```python
from build123d import *

# Parameters (mm, degrees)
BOSS_EXTRUDE1_DEPTH     = 15
SCALE1_SCALE            = 0.6
CUT_EXTRUDE2_DEPTH      = 414.628802078
CUT_EXTRUDE2_DEPTH_BACK = 414.628802078


with BuildPart() as part:
    # Sketch3 → Boss-Extrude1 (new body)
    with BuildSketch(Plane.XY):
        Polygon((373.374123275, 416.968077367), (402.437373481, 34.910153282), (374.539751445, 1.298077367), (346.074948764, 1.298077367), (346.074948764, 416.968077367), align=None)
    extrude(amount=BOSS_EXTRUDE1_DEPTH)


with BuildPart() as part_1:
    # Scale1: scaled about (367.849283485, 188.760033588, 7.5)
    add(part.part.scale(SCALE1_SCALE).moved(Location((147.139713394, 75.504013435, 3))))

    # Sketch9 → Cut-Extrude2 (cut, two sides: drawn at the far end of the back side and taken through both)
    with BuildSketch(Plane(origin=(0, 184.5, 0), x_dir=(1, 0, 0), z_dir=(0, 1, 0)).offset(-CUT_EXTRUDE2_DEPTH_BACK)):
        with BuildLine():
            Line((354.784682653, -12), (354.784682653, -3))
            ThreePointArc((354.784682653, -3), (356.648643683, -7.5), (354.784682653, -12))
        make_face()
    extrude(amount=CUT_EXTRUDE2_DEPTH + CUT_EXTRUDE2_DEPTH_BACK, mode=Mode.SUBTRACT)


solid = part_1.part
```
The listing builds one solid part. Answer for the finished solid, in the listing's coordinates (mm). Round coordinates to 2 decimals unless told otherwise and drop trailing zeros. Order: outer loops, then holes, each group sorted by start corner. A loop starts at its lowest first (then second) coordinate and runs counter-clockwise, first axis right, second up. Notation, with made-up numbers: (47, -22) -> (55, -22) arc R12 ccw to (55, -5) -> close; hole circle Ø8 at (-26.75, -10). An arc over 180 degrees is marked (long way). Answer as CSV lines item,"result". Start each with the question number.
(1) Find the intervals of material crossed by probe 1 along X at (y, z) = (130, 8.5); probe 2 along X at (y, z) = (311.5, 4.75), in increasing order. Write a range as from..to.
(2) Flat-ended cylindrical pins translate along their axes: pin 1 Ø4 at (y, z) = (177.5, 6) entering from -X; pin 2 Ø1 at (y, z) = (238.5, 5) entering from +X; pin 3 Ø1.5 at (y, z) = (200.5, 4.5) entering from +X. Find the tip coordinate at first contact, or state that the pin passes through.
(3) For a pull along Z with two mould halves and no side action, classify faces 1 (the face through (368, 203, 12)), 2 (the face through (379.76, 212.67, 7.44)), 3 (the face through (356.65, 199.24, 7.43)) as +Z half, -Z half, draft (parallel to the pull), parting line (faces both ways), or undercut.
(4) The part is cut by section C-C (x = 385.5). Determine the outline of the cut face in (y, z), then the cut area to 3 significant figures.
(5) The part is cut by section B-B (y = 238.5). Determine the outline of the cut face in (x, z).
(6) The part is cut by section A-A (z = 4.5). Determine the outline of the cut face in (x, y), then the cut area to 3 significant figures.
Evaluation:
1,probe 1,"356.57..386.05"
1,probe 2,"356.02..372.24"
2,pin 1,"x = 355.6"
2,pin 2,"x = 377.83"
2,pin 3,"x = 380.74"
3,face 1,"+Z half"
3,face 2,"draft"
3,face 3,"undercut"
4,outline,"(92.71, 3) -> (137.23, 3) -> (137.23, 12) -> (92.71, 12) -> close"
4,area,"401 mm²"
5,outline,"(354.78, 3) -> (377.8, 3) -> (377.8, 12) -> (354.78, 12) arc R6.36 cw to start"
6,outline,"(355.9, 76.28) -> (371.86, 76.28) -> (388.6, 96.45) -> (371.16, 325.68) -> (355.9, 325.68) -> close"
6,area,"5,990 mm²"
